Geometry check sheet. Reference: drawing and pictorial views, mm from the part's lowest x, y, z. Give positions to 0.01 mm unless a question says otherwise; leave off trailing zeros. Order: outer loops, then holes, each group sorted by start corner. A loop starts at its lowest first (then second) coordinate and runs counter-clockwise, first axis right, second up.
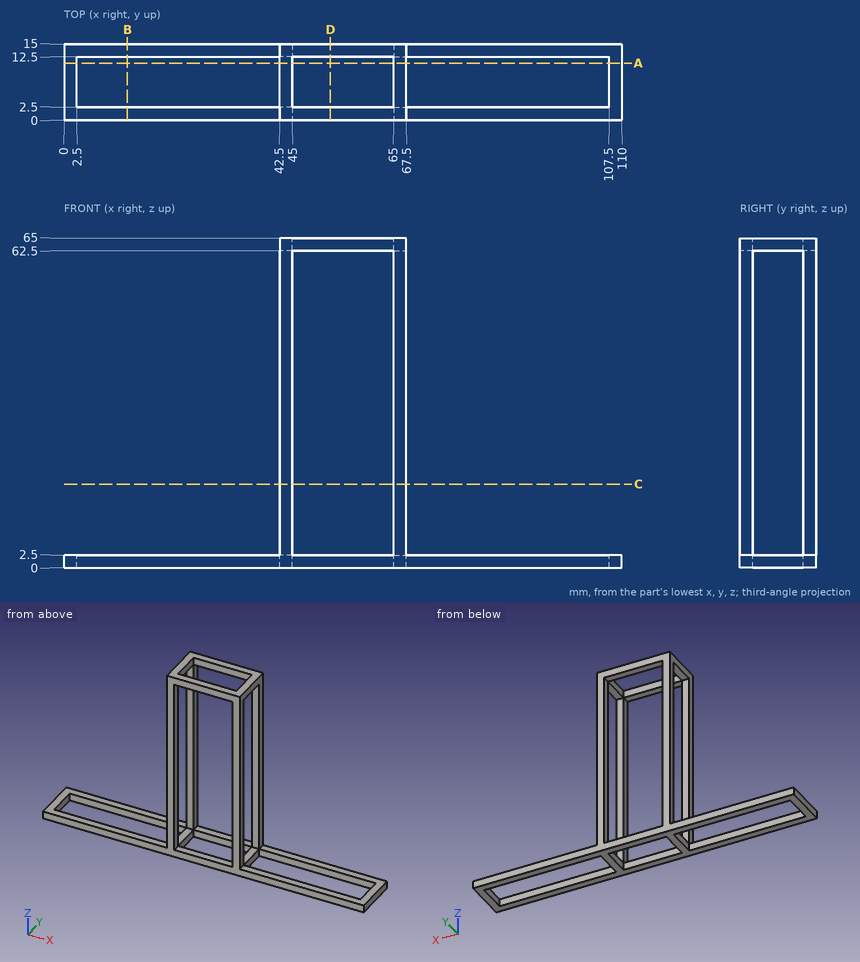
1) Section check C-C, the plane z = 16.5. Record the cut outline in (x, y), then the cut area to 3 significant figures.
Recorded:
outline: (42.5, 0) - (45, 0) - (45, 2.5) - (42.5, 2.5) - close; (42.5, 12.5) - (45, 12.5) - (45, 15) - (42.5, 15) - close; (65, 0) - (67.5, 0) - (67.5, 2.5) - (65, 2.5) - close; (65, 12.5) - (67.5, 12.5) - (67.5, 15) - (65, 15) - close
area: 25.0 mm2
2) Section check A-A, the plane y = 11.25. Record the cut outline in (x, z).
Recorded:
outline: (0, 0) - (2.5, 0) - (2.5, 2.5) - (0, 2.5) - close; (42.5, 0) - (45, 0) - (45, 2.5) - (42.5, 2.5) - close; (42.5, 62.5) - (45, 62.5) - (45, 65) - (42.5, 65) - close; (65, 0) - (67.5, 0) - (67.5, 2.5) - (65, 2.5) - close; (65, 62.5) - (67.5, 62.5) - (67.5, 65) - (65, 65) - close; (107.5, 0) - (110, 0) - (110, 2.5) - (107.5, 2.5) - close
3) Section check D-D, the plane x = 52.5. Record the cut outline in (y, z), then the cut area to 3 significant figures.
Recorded:
outline: (0, 0) - (2.5, 0) - (2.5, 2.5) - (0, 2.5) - close; (0, 62.5) - (2.5, 62.5) - (2.5, 65) - (0, 65) - close; (12.5, 0) - (15, 0) - (15, 2.5) - (12.5, 2.5) - close; (12.5, 62.5) - (15, 62.5) - (15, 65) - (12.5, 65) - close
area: 25.0 mm2
4) Depth check by flat-ended pin: pin 1 Ø4 at (y, z) = (12, 35) entering from -X; pin 2 Ø5 at (y, z) = (5.5, 55) entering from +X; pin 3 Ø1.2 at (y, z) = (1.5, 24) entering from +X. Enter the tip coordinate at first touch or a pass-through.
Recorded:
pin 1: stops at x = 42.5
pin 2: passes through
pin 3: stops at x = 67.5
5) Section check B-B, the plane x = 12.5. Record the cut outline in (y, z).
Recorded:
outline: (0, 0) - (2.5, 0) - (2.5, 2.5) - (0, 2.5) - close; (12.5, 0) - (15, 0) - (15, 2.5) - (12.5, 2.5) - close
6) Material ranges on L1, parallel to Z at x = 54, y = 1; L2, parallel to Y at x = 43.5, z = 48.5; L3, parallel to X at y = 2.25, z = 27.5, recorded low to high.
Recorded:
L1: z = 0 to 2.5, 62.5 to 65
L2: y = 0 to 2.5, 12.5 to 15
L3: x = 42.5 to 45, 65 to 67.5
